from build123d import *

# Parameters (mm, degrees)
F1_DEPTH = 12.7
F2_SIZE  = 3.81
F3_R     = 1.27
F4_DEPTH = 7.62


with BuildPart() as f1:
    # F0 (on Front) → F1 (new body, symmetric)
    with BuildSketch(Plane.XZ):
        with BuildLine():
            Line((0, -25.4), (0, 25.4))
            ThreePointArc((0, 25.4), (-1.8598719395, 29.8901280605), (-6.35, 31.75))
            Line((-6.35, 31.75), (-57.15, 31.75))
            Line((-57.15, 31.75), (-57.15, 22.86))
            Line((-57.15, 22.86), (-11.43, 22.86))
            ThreePointArc((-11.43, 22.86), (-9.6339487758, 22.1160512242), (-8.89, 20.32))
            Line((-8.89, 20.32), (-8.89, -25.4))
            Line((-8.89, -25.4), (0, -25.4))
        make_face()
    extrude(amount=F1_DEPTH, both=True)

    # F2
    f2_edges = [f1.edges().sort_by_distance(p)[0] for p in [
        (-31.75, -12.7, 31.75),
        (-34.29, -12.7, 22.86),
    ]]
    chamfer(f2_edges, length=F2_SIZE)

    # F3 (on face) → F4 (cut)
    with BuildSketch(Plane(origin=(-8.89, 0, 0), x_dir=(0, -1, 0), z_dir=(-1, 0, 0))):
        with Locations((-1.905, 3.81)):
            Circle(F3_R)
    extrude(amount=-F4_DEPTH, mode=Mode.SUBTRACT)


solid = f1.part
Can you work these out from the model? Positions are in its coordinate system, mm. A direction names the side the tool comes from. Coordinates: 2 decimals unless noted, no trailing zeros. Loops run counter-clockwise (first coordinate to the right, second up) from the corner with the lowest first, then second, coordinate; pieces in that order, holes last. Notation, with made-up numbers: M 69,-23 L 96,-23 A27 cw 96,1 Z; hole C -10.75,-20.75 d8. An arc over 180 degrees is marked long. Return JSON: item names as keys, results as strings. Group by question number.
Item 1: Imagine slicing it at A-A (y = 8.5). Please give me the cut outline in (x, z).
Item 2: Imagine slicing it at C-C (z = 17). Please give me the cut outline in (x, y).
Item 3: On a 3-axis mill with a long thin cutter (end or side, diameter ignored), from which of +Z, -Z, +X, -X, +Y, -Y can I reach the whole of each face in a straight line? I mean faces 4 (the flat face through (-6.96, -10.82, -2.22)), 5 (the cylindrical face through (-5.13, 2.18, 2.57)), 6 (the conical face through (-3, -11, 28)), 7 (the flat face through (-35, 2, 22.86)), 8 (the flat face through (-8, 12.7, 14)). Say none if no direction works.
Item 4: Imagine slicing it at B-B (x = -47). Please give me the cut outline in (y, z), and give its area (3 significant figures).
Item 5: Imagine slicing it at D-D (z = 3.81). Please give me the cut outline in (x, y) (3 decimals), and give its area (3 significant figures).
Item 6: If I drill on L1, parallel to X at y = 10.5, z = -20; L2, parallel to Z at x = -20.5, y = 2; L3, parallel to Y at x = -3, z = 3, over which ranges is the centre line in solid material (lowest first)? Write a range as from..to.
Item 7: I'm going to push flat-ended pins straight in: pin 1 Ø6 at (x, y) = (-16, -1.5) entering from -Z; pin 2 Ø2 at (y, z) = (1.905, 3.81) entering from -X; pin 3 Ø1 at (y, z) = (7.5, -0.5) entering from -X. Where does each tip first touch, or does it pass through?
Item 8: Thinking about a two-plate mould opening in Z: for faces 1 (the flat face through (-1.27, 2, 4)), 2 (the flat face through (-8.89, 2, -2)), 3 (the cylindrical face through (-1.81, 1.75, 29.84)), which applies, released by +Z, released by -Z, zero draft, split by the parting line, or undercut?
Verdict:
{
 "1": {"outline": "M -57.15,22.86 L -11.43,22.86 A2.54 cw -8.89,20.32 L -8.89,-25.4 L 0,-25.4 L 0,25.4 A6.35 ccw -6.35,31.75 L -57.15,31.75 Z"},
 "2": {"outline": "M -8.89,-8.89 L -5.08,-12.7 L -3.81,-12.7 L 0,-8.89 L 0,12.7 L -8.89,12.7 Z"},
 "3": {"face 4": "-Z, -X, -Y", "face 5": "-X", "face 6": "+Z, +X, -Y", "face 7": "-Z, -X, +Y, -Y", "face 8": "+Z, -Z, +X, -X, +Y"},
 "4": {"outline": "M -12.7,26.67 L -8.89,22.86 L 12.7,22.86 L 12.7,31.75 L -8.89,31.75 L -12.7,27.94 Z", "area": "211 mm^2"},
 "5": {"outline": "M -8.89,-8.89 L -5.08,-12.7 L -3.81,-12.7 L 0,-8.89 L 0,12.7 L -8.89,12.7 L -8.89,3.175 L -1.27,3.175 L -1.27,0.635 L -8.89,0.635 Z", "area": "192 mm^2"},
 "6": {"L1": "x = -8.89..0", "L2": "z = 22.86..31.75", "L3": "y = -11.89..0.93, 2.88..12.7"},
 "7": {"pin 1": "stops at z = 22.86", "pin 2": "stops at x = -1.27", "pin 3": "stops at x = -8.89"},
 "8": {"face 1": "undercut", "face 2": "zero draft", "face 3": "released by +Z"}
}
